Geometry check sheet. Reference: drawing and pictorial views, mm from the part's lowest x, y, z. A direction names the side the tool comes from. Give positions to 0.01 mm unless a question says otherwise; leave off trailing zeros. Order: outer loops, then holes, each group sorted by start corner. A loop starts at its lowest first (then second) coordinate and runs counter-clockwise, first axis right, second up. Notation, with made-up numbers: (-17.5, -3) - (23.5, -3) arc R22 ccw to (23.5, 25) - close; hole circle Ø10 at (5.5, -40). An arc over 180 degrees is marked (long way). Answer as a JSON object with one key per item and string values.
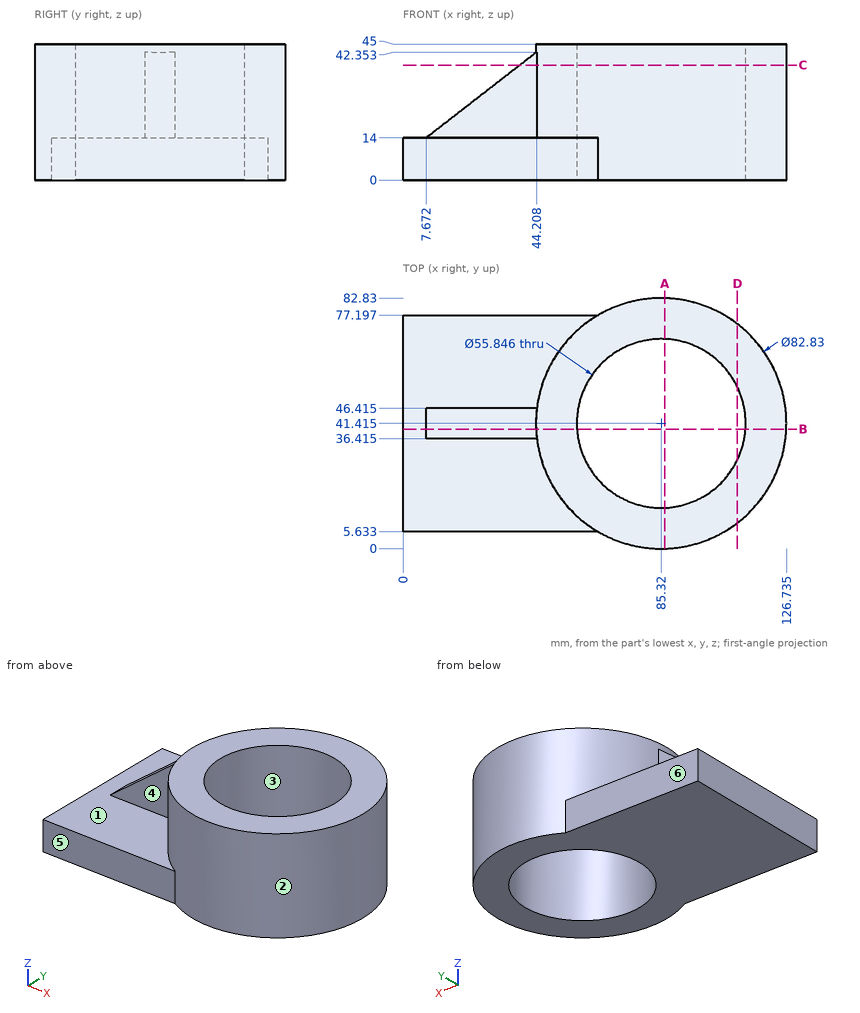
(1) Section check B-B (y = 39.5). Record the cut outline in (x, z), then the cut area to 3 significant figures.
Computed values:
{"outline": "(0, 0) - (57.46, 0) - (57.46, 45) - (43.95, 45) - (43.95, 42.15) - (7.67, 14) - (0, 14) - close; (113.18, 0) - (126.69, 0) - (126.69, 45) - (113.18, 45) - close", "area": "2,340 mm²"}
(2) Section check C-C (z = 38). Record the cut outline in (x, y) (1 decimal), then the cut area to 3 significant figures.
Computed values:
{"outline": "(38.6, 36.4) - (44.2, 36.4) arc R41.4 ccw (long way) to (44.2, 46.4) - (38.6, 46.4) - close; hole circle Ø55.8 at (85.3, 41.4)", "area": "2,990 mm²"}
(3) Material ranges on line 1 along Z through (x, y) = (14, 64); line 2 along Y through (x, z) = (43.5, 24) (1 decimal); line 3 along X through (y, z) = (16.5, 33) (1 decimal), recorded low to high. Write a range as [from, to].
Computed values:
{"line 1": "z = [0, 14]", "line 2": "y = [36.4, 46.4]", "line 3": "x = [52.2, 72.7], [97.9, 118.4]"}
(4) Section check D-D (x = 110.5). Record the cut outline in (y, z) (1 decimal), then the cut area to 3 significant figures.
Computed values:
{"outline": "(8.5, 0) - (29.3, 0) - (29.3, 45) - (8.5, 45) - close; (53.5, 0) - (74.3, 0) - (74.3, 45) - (53.5, 45) - close", "area": "1,870 mm²"}
(5) Release check for a two-part mould opening along X. For the marked faces 1, 2 and 3 record: pulls with the +X half, pulls with the -X half, needs draft (parallel to the pull), parting line crosses it, or undercut.
Computed values:
{"face 1": "needs draft", "face 2": "parting line crosses it", "face 3": "undercut"}
(6) Access from +Z, -Z, +X, -X, +Y, -Y to the whole of each face (thin tool, end or side, straight path). Record for the marked faces 4, 5 and 6.
Computed values:
{"face 4": "+Z, -X, -Y", "face 5": "+Z, -Z, -X, -Y", "face 6": "+Z, -Z, -X, +Y"}
(7) Gauge pin test, flat ends, axial feed: pin 1 Ø3 at (x, z) = (111.5, 30.5) entering from -Y; pin 2 Ø4 at (x, z) = (65.5, 7) entering from +Y; pin 3 Ø8 at (x, z) = (33.5, 7) entering from +Y; pin 4 Ø8 at (x, y) = (109, 20.5) entering from -Z. Record the tip position at first contact, or that the pin passes through.
Computed values:
{"pin 1": "stops at y = 8.16", "pin 2": "stops at y = 78.8", "pin 3": "stops at y = 77.2", "pin 4": "stops at z = 0"}
(8) Section check A-A (x = 86.5). Record the cut outline in (y, z), then the cut area to 4 significant figures.
Computed values:
{"outline": "(0.02, 0) - (13.52, 0) - (13.52, 45) - (0.02, 45) - close; (69.31, 0) - (82.81, 0) - (82.81, 45) - (69.31, 45) - close", "area": "1,215 mm²"}
